Part print with two shaded views. Sizes in mm from the minimum x, y, z corner. A direction names the side the tool comes from. Round coordinates to 2 decimals unless told otherwise and drop trailing zeros. Loops run counter-clockwise (first coordinate to the right, second up) from the corner with the lowest first, then second, coordinate; pieces in that order, holes last. Notation, with made-up numbers: M 19,-31 L 62,-31 A21 ccw 62,2 Z; hole C 12,70.5 d7. An arc over 180 degrees is marked long. Answer as CSV lines item,"result". Start each with the question number.
Item 1: Band-saw the part on A-A (x = 3). Give the cut face in (y, z), and give its area (3 significant figures).
Item 2: Band-saw the part on B-B (z = 9.25). Give the cut face in (x, y).
Item 3: Drop flat-ended pins along their axis: pin 1 Ø0.6 at (x, z) = (3.5, 1) entering from +Y; pin 2 Ø3 at (x, z) = (1.5, 11) entering from +Y; pin 3 Ø0.9 at (x, z) = (3, 0.5) entering from -Y. Give the stop position or say it passes through.
Item 4: Which spindle directions (+Z, -Z, +X, -X, +Y, -Y) get a long thin tool onto all of the face, cutting with end or side? Do the marked faces 1, 2 and 3. Say none if no direction does.
Item 5: Wall check: line 1 (Y direction, x = 2.25, z = 4.25); line 2 (Z direction, x = 3.8, y = 3.45); line 3 (X direction, y = 3.85, z = 12.25) (1 decimal). Give the ranges that are in metal, low to high.
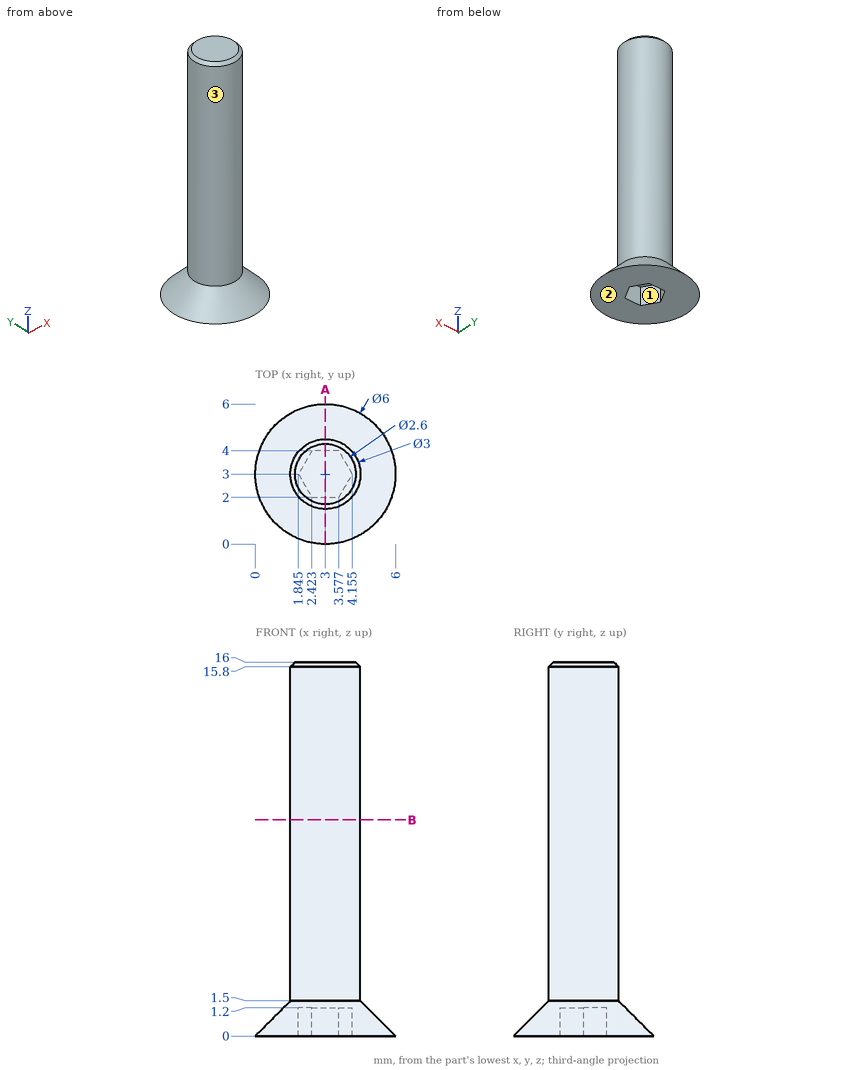
Answer block:
1,outline,"M 0,0 L 2,0 L 2,1.2 L 4,1.2 L 4,0 L 6,0 L 4.5,1.5 L 4.5,15.8 L 4.3,16 L 1.7,16 L 1.5,15.8 L 1.5,1.5 Z"
1,area,"47.8 mm^2"
2,outline,"C 3,3 d3"
3,pin 1,"stops at y = 5.25"
3,pin 2,"stops at y = 4.5"
3,pin 3,"stops at y = 0.05"
4,face 1,"-Z"
4,face 2,"-Z, +X, -X, +Y, -Y"
4,face 3,"+Z"
5,line 1,"y = 1.7 to 4.3"
5,line 2,"z = 1.2 to 16"
5,line 3,"x = 1.8 to 4.2"
